Could you check a few things on this model? Use its own coordinates, in mm. Face numbers are marked on the shaded views. Give positions to 0.01 mm unless a question says otherwise; leave off trailing zeros. Loops run counter-clockwise (first coordinate to the right, second up) from the corner with the lowest first, then second, coordinate; pieces in that order, holes last. Notation, with made-up numbers: M 80,76 L 134,76 A20 ccw 134,111 Z; hole C 80,11.25 d1. An arc over 180 degrees is marked long. Return JSON: item names as keys, results as strings. Group by question number.
1. For pin 1 (1.5 mm diameter, centred on x = -1.5, y = 7.5, fed in from +Z); pin 2 (1 mm diameter, centred on x = -1, z = 0.5, fed in from +Y); pin 3 (3 mm diameter, centred on x = 3.5, y = 2.5, fed in from +Z), each with a flat end and sliding along its axis, tell me the tip position at first contact or that it passes through.
2. Please list where these lines run through material, in increasing order: line 1 (X direction, y = 4, z = 1.25); line 2 (Z direction, x = 0.25, y = 3); line 3 (X direction, y = 1, z = 0.75).
3. If we mould it in two halves opening along Z, with no side actions, what happens to the marked faces 1, 2, 3 and 4? For each: +Z half, -Z half, draft (parallel to the pull), parting line (faces both ways), or undercut.
4. If we section it at A-A (y = 3): Write out the boundary of the cut face in (x, z) (3 decimals), plus the area to 3 significant figures.
5. If we section it at B-B (y = 5.5): Write out the boundary of the cut face in (x, z).
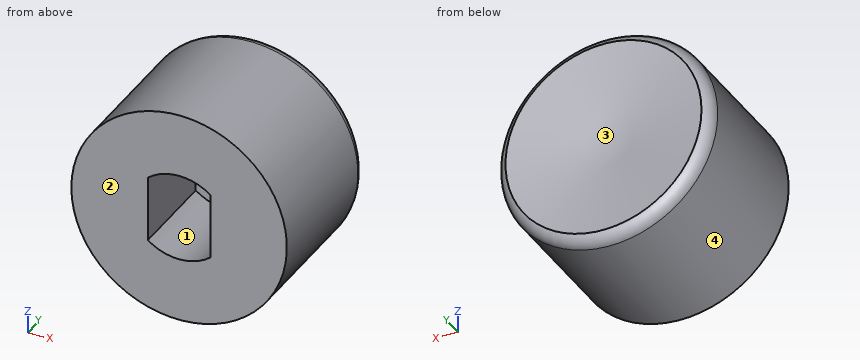
```python
from build123d import *

# Parameters (mm, degrees)
F3_DEPTH = 5.334


with BuildPart() as f1:
    # F0 (on Top) → F1 (revolve)
    with BuildSketch(Plane.XY):
        with BuildLine():
            Line((-6.223, 0), (0, 0))
            Line((0, 0), (0, 7.874))
            Line((0, 7.874), (-5.659229, 8.636))
            ThreePointArc((-5.659229, 8.636), (-6.037134, 8.351132), (-6.223, 7.915913))
            Line((-6.223, 7.915913), (-6.223, 0))
        make_face()
    revolve(axis=Axis((0, 3.937, 0), (0, -1, 0)))

    # F2 (on Front) → F3 (cut)
    with BuildSketch(Plane.XZ):
        with BuildLine():
            Line((1.8034, -1.905), (1.8034, 1.905))
            ThreePointArc((1.8034, 1.905), (0, 2.538774), (-1.8034, 1.905))
            Line((-1.8034, 1.905), (-1.8034, -1.905))
            ThreePointArc((-1.8034, -1.905), (0, -2.538774), (1.8034, -1.905))
        make_face()
    extrude(amount=-F3_DEPTH, mode=Mode.SUBTRACT)


solid = f1.part
```
Answer:
{
 "1": {"pin 1": "stops at z = 6.18", "pin 2": "stops at y = 8.09", "pin 3": "stops at z = 5.89"},
 "2": {"line 1": "x = -6.1 to -1.8, 1.8 to 6.1", "line 2": "z = -6.22 to -2.53, 2.53 to 6.22", "line 3": "x = -6.18 to -1.8, 1.8 to 6.18"},
 "3": {"face 1": "undercut", "face 2": "draft", "face 3": "undercut", "face 4": "parting line"},
 "4": {"outline": "C 0,0 d12.446; hole M -1.803,-1.905 A2.883 ccw 1.803,-1.905 L 1.803,1.905 A2.883 ccw -1.803,1.905 Z", "area": "105 mm²"},
 "5": {"outline": "C 0,0 d12.45"}
}
